Part model, mm, in its own coordinate system. Round coordinates to 2 decimals unless told otherwise and drop trailing zeros. Order: outer loops, then holes, each group sorted by start corner. A loop starts at its lowest first (then second) coordinate and runs counter-clockwise, first axis right, second up. Notation, with made-up numbers: (85.25, -25.5) -> (92.25, -25.5) arc R35 ccw to (92.25, 13.5) -> close; hole circle Ø10 at (76, -36). An arc over 180 degrees is marked (long way). Answer as a JSON object with one key per item and string values. Group by question number.
Autodesk Inventor part; units mm, degrees
ref_plane "YZ Plane" through (0, 0, 0) normal (1, 0, 0) x (0, 1, 0)
ref_plane "XZ Plane" through (0, 0, 0) normal (0, 1, 0) x (-1, 0, 0)
ref_plane "XY Plane" through (0, 0, 0) normal (0, 0, 1) x (1, 0, 0)
sketch "Sketch1" plane through (0, 0, 0) normal (0, 1, 0) x (-1, 0, 0)
  line L0 (0, 0) -> (60, 0)
  line L1 (60, 0) -> (60, -4)
  line L2 (60, -4) -> (0, -4)
  line L3 (0, -4) -> (0, 0)
  dimension "d0" = 60
  dimension "d1" = 4
extrude "Extrusion1" add sketch "Sketch1" along normal blind 4
sketch "Sketch2" plane through (0, 4, 0) normal (0, 1, 0) x (1, 0, 0)
  line L0 (0, 0) -> (0, 4)
  line L1 (0, 2) -> (-2, 2)
  circle A0 centre (-2, 2) radius 1
  line L2 (0, 4) -> (-60, 4)
  line L3 (-30, 4) -> (-30, 1.3223)
  circle A1 centre (-58, 2) radius 1
  dimension "d4" = 2
  dimension "d5" = 2
extrude "Extrusion2" cut sketch "Sketch2" against normal blind 4
sketch "Sketch3" plane through (0, 4, 0) normal (0, 1, 0) x (1, 0, 0)
  line L0 (0, 0) -> (0, 4)
  line L1 (0, 2) -> (-60, 2)
  line L2 (-60, 4) -> (-60, 0)
  circle A0 centre (-30, 2) radius 1
  circle A1 centre (-27, 2) radius 1
  circle A2 centre (-33, 2) radius 1
  circle A3 centre (-30, 2) radius 1
  dimension "d8" = 2
  dimension "d13" = 3
  dimension "d16" = 3
extrude "Extrusion3" cut sketch "Sketch3" against normal blind 10 contours A0 L1 | L1 A0
extrude "Extrusion4" cut sketch "Sketch3" against normal blind 10 contours A1 L1 | L1 A1 | A2 L1 | L1 A2
properties part number "parallel_bar_long_v1"
Q1. Two-plate mould, pull along Z, no slides. Class faces 1 (the flat face through (-29.6, 4, -0.6)), 2 (the flat face through (-30, 2, 0)), 3 (the cylindrical face through (-29, 2, -2)): +Z half, -Z half, draft (parallel to the pull), parting line (faces both ways), or undercut.
Q2. Band-saw the part on C-C (x = -2). List the corners of the cut face in (y, z), plus the area to 3 significant figures.
Q3. Wall check: line 1 (X direction, y = 2.7, z = -2); line 2 (X direction, y = 1.5, z = -1.35); line 3 (Z direction, x = -58, y = 2.95). Give the ranges that are in metal, low to high. Write a range as [from, to].
Q4. Band-saw the part on A-A (z = -2). List the corners of the cut face in (x, y), plus the area to 3 significant figures.
Q5. Band-saw the part on B-B (y = 1.6). List the corners of the cut face in (x, z).
Completed:
{
 "1": {"face 1": "draft", "face 2": "+Z half", "face 3": "undercut"},
 "2": {"outline": "(0, -4) -> (4, -4) -> (4, -3) -> (0, -3) -> close; (0, -1) -> (4, -1) -> (4, 0) -> (0, 0) -> close", "area": "8.00 mm2"},
 "3": {"line 1": "[-60, -59], [-57, -34], [-32, -31], [-29, -28], [-26, -3], [-1, 0]", "line 2": "[-60, -58.76], [-57.24, -33.76], [-32.24, -30.76], [-29.24, -27.76], [-26.24, -2.76], [-1.24, 0]", "line 3": "[-4, -3], [-1, 0]"},
 "4": {"outline": "(-60, 0) -> (-59, 0) -> (-59, 4) -> (-60, 4) -> close; (-57, 0) -> (-34, 0) -> (-34, 4) -> (-57, 4) -> close; (-32, 0) -> (-31, 0) -> (-31, 4) -> (-32, 4) -> close; (-29, 0) -> (-28, 0) -> (-28, 4) -> (-29, 4) -> close; (-26, 0) -> (-3, 0) -> (-3, 4) -> (-26, 4) -> close; (-1, 0) -> (0, 0) -> (0, 4) -> (-1, 4) -> close", "area": "200 mm2"},
 "5": {"outline": "(-60, -4) -> (0, -4) -> (0, 0) -> (-60, 0) -> close; hole circle Ø2 at (-58, -2); hole circle Ø2 at (-33, -2); hole circle Ø2 at (-30, -2); hole circle Ø2 at (-27, -2); hole circle Ø2 at (-2, -2)"}
}
